Geometry: see drawing. Coordinates: mm, zero at the bounding-box minimum. A direction names the side the tool comes from. Give positions to 0.01 mm unless a question says otherwise; leave off trailing zeros. Loops run counter-clockwise (first coordinate to the right, second up) from the corner with the lowest first, then second, coordinate; pieces in that order, holes last. Notation, with made-up numbers: M -2.5,-38 L 31.5,-38 A33 ccw 31.5,-3 Z; hole C 27,34 d10. An arc over 180 degrees is marked long. Answer in a Markdown table with one row per item.
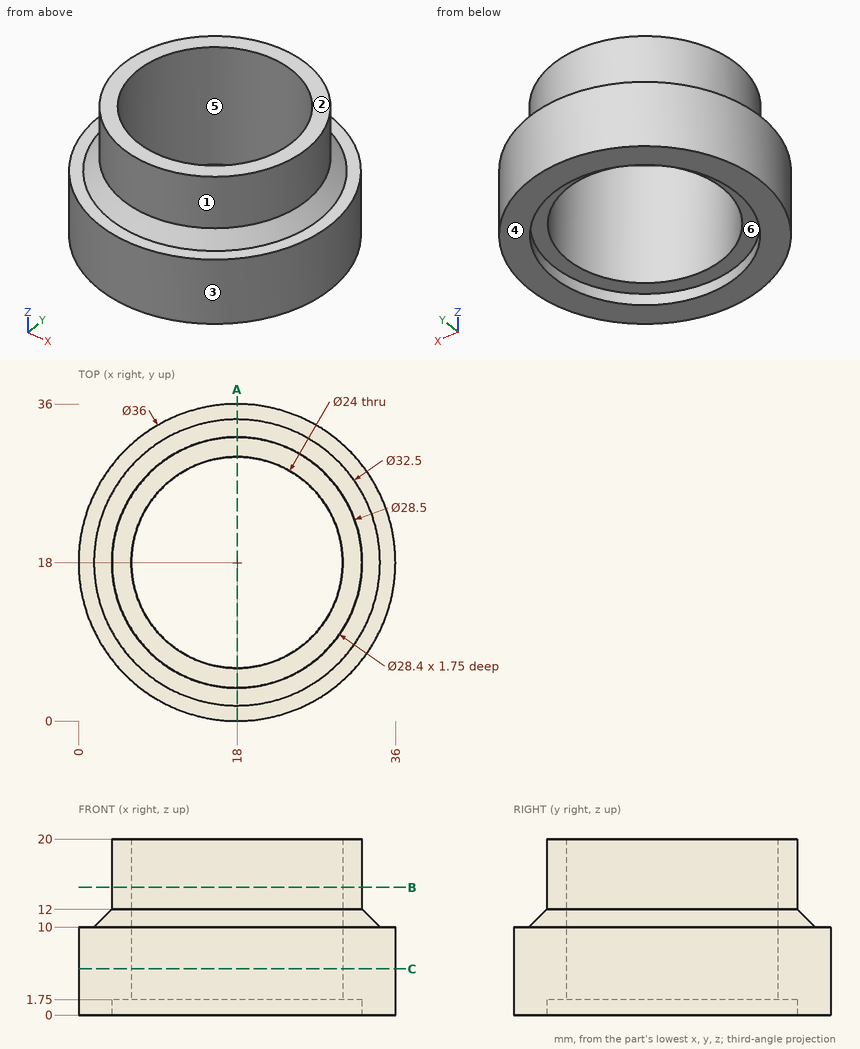
1) Section B-B, the plane z = 14.5. Return loops of the section in (x, y), then the cut area to 3 significant figures.
Reply:
| item | result |
|---|---|
| outline | C 18,18 d28.5; hole C 18,18 d24 |
| area | 186 mm² |
2) Pull-direction query (Y, two-part tool) for the marked faces 3, 4, 5 and 6; classes: released by +Y, released by -Y, zero draft, split by the parting line, or undercut.
Reply:
| item | result |
|---|---|
| face 3 | split by the parting line |
| face 4 | zero draft |
| face 5 | undercut |
| face 6 | undercut |
3) Section C-C, the plane z = 5.25. Return loops of the section in (x, y).
Reply:
| item | result |
|---|---|
| outline | C 18,18 d36; hole C 18,18 d24 |
4) Section A-A, the plane x = 18. Return loops of the section in (y, z).
Reply:
| item | result |
|---|---|
| outline | M 0,0 L 3.8,0 L 3.8,1.75 L 6,1.75 L 6,20 L 3.75,20 L 3.75,12 L 1.75,10 L 0,10 Z; M 30,1.75 L 32.2,1.75 L 32.2,0 L 36,0 L 36,10 L 34.25,10 L 32.25,12 L 32.25,20 L 30,20 Z |
5) Pin query (flat end, axial travel): pin 1 Ø2 at (x, z) = (22.5, 7.5) entering from +Y; pin 2 Ø8 at (x, y) = (26.5, 7) entering from -Z; pin 3 Ø12 at (x, z) = (14, 15.5) entering from +Y; pin 4 Ø14 at (x, y) = (21.5, 15) entering from -Z. Return the tip coordinate at first contact, or that it passes through.
Reply:
| item | result |
|---|---|
| pin 1 | stops at y = 35.66 |
| pin 2 | stops at z = 0 |
| pin 3 | stops at y = 35.93 |
| pin 4 | passes through |
6) Material intervals for L1, parallel to Y at x = 18, z = 0.75; L2, parallel to Y at x = 18, z = 9.25; L3, parallel to X at y = 16, z = 4.5, sorted ascending.
Reply:
| item | result |
|---|---|
| L1 | y = 0 to 3.8, 32.2 to 36 |
| L2 | y = 0 to 6, 30 to 36 |
| L3 | x = 0.11 to 6.17, 29.83 to 35.89 |
7) Set-up query: the marked faces 1 and 2. Return all of +Z, -Z, +X, -X, +Y, -Y with unobstructed straight access to the full face (end or side cutting, diameter ignored); none if empty.
Reply:
| item | result |
|---|---|
| face 1 | +Z |
| face 2 | +Z, +X, -X, +Y, -Y |
